Check sheet for the modelled part. Datum: model origin and axes. Units: mm. A direction names the side the tool comes from. Coordinates: 2 decimals unless noted, no trailing zeros. Loops run counter-clockwise (first coordinate to the right, second up) from the corner with the lowest first, then second, coordinate; pieces in that order, holes last.
```python
from build123d import *

# Parameters (mm, degrees)
SKETCH1_R                    = 254
BOSS_EXTRUDE1_DEPTH          = 2.54
SKETCH2_R                    = 228.6
SKETCH2_R_2                  = 226.06
CUT_EXTRUDE1_DEPTH           = 1.27
CUT_EXTRUDE2_DEPTH           = 1.27
SKETCH8_R                    = 6.35
CUT_EXTRUDE3_DEPTH           = 360.219224987
F_10_0_1935_DIAMETER_HOLE1_D = 4.9149


with BuildPart() as part:
    # Sketch1 → Boss-Extrude1 (new body)
    with BuildSketch(Plane.XY):
        Circle(SKETCH1_R)
    extrude(amount=BOSS_EXTRUDE1_DEPTH)

    # Sketch2 → Cut-Extrude1 (cut)
    with BuildSketch(Plane.XY.offset(2.54)):
        Circle(SKETCH2_R)
        Circle(SKETCH2_R_2, mode=Mode.SUBTRACT)
    extrude(amount=-CUT_EXTRUDE1_DEPTH, mode=Mode.SUBTRACT)

    # Sketch4 → Cut-Extrude2 (cut)
    with BuildSketch(Plane.XY.offset(2.54)):
        with BuildLine():
            Line((-226.06, 0), (-175.26, 18.489687901))
            Line((-175.26, 18.489687901), (-176.128731164, 20.876507158))
            Line((-176.128731164, 20.876507158), (-226.043768674, 2.708919262))
            ThreePointArc((-226.043768674, 2.708919262), (-226.055942132, 1.354483944), (-226.06, 0))
        make_face()
        with BuildLine():
            Line((-195.77370278, 113.03), (-142.534768317, 103.64253943))
            Line((-142.534768317, 103.64253943), (-142.093701946, 106.143951123))
            Line((-142.093701946, 106.143951123), (-194.405186408, 115.367877234))
            ThreePointArc((-194.405186408, 115.367877234), (-195.092946591, 114.200988571), (-195.77370278, 113.03))
        make_face()
        with BuildLine():
            Line((-113.03, 195.77370278), (-71.61746057, 161.024456218))
            Line((-71.61746057, 161.024456218), (-69.984780041, 162.970209103))
            Line((-69.984780041, 162.970209103), (-110.67589144, 197.11410567))
            ThreePointArc((-110.67589144, 197.11410567), (-111.854953561, 196.447430535), (-113.03, 195.77370278))
        make_face()
        with BuildLine():
            Line((0, 226.06), (18.489687901, 175.26))
            Line((18.489687901, 175.26), (20.876507158, 176.128731164))
            Line((20.876507158, 176.128731164), (2.708919262, 226.043768674))
            ThreePointArc((2.708919262, 226.043768674), (1.354483944, 226.055942132), (0, 226.06))
        make_face()
        with BuildLine():
            Line((113.03, 195.77370278), (103.64253943, 142.534768317))
            Line((103.64253943, 142.534768317), (106.143951123, 142.093701946))
            Line((106.143951123, 142.093701946), (115.367877234, 194.405186408))
            ThreePointArc((115.367877234, 194.405186408), (114.200988571, 195.092946591), (113.03, 195.77370278))
        make_face()
        with BuildLine():
            Line((195.77370278, 113.03), (161.024456218, 71.61746057))
            Line((161.024456218, 71.61746057), (162.970209103, 69.984780041))
            Line((162.970209103, 69.984780041), (197.11410567, 110.67589144))
            ThreePointArc((197.11410567, 110.67589144), (196.447430535, 111.854953561), (195.77370278, 113.03))
        make_face()
        with BuildLine():
            Line((226.06, 0), (175.26, -18.489687901))
            Line((175.26, -18.489687901), (176.128731164, -20.876507158))
            Line((176.128731164, -20.876507158), (226.043768674, -2.708919262))
            ThreePointArc((226.043768674, -2.708919262), (226.055942132, -1.354483944), (226.06, 0))
        make_face()
        with BuildLine():
            Line((195.77370278, -113.03), (142.534768317, -103.64253943))
            Line((142.534768317, -103.64253943), (142.093701946, -106.143951123))
            Line((142.093701946, -106.143951123), (194.405186408, -115.367877234))
            ThreePointArc((194.405186408, -115.367877234), (195.092946591, -114.200988571), (195.77370278, -113.03))
        make_face()
        with BuildLine():
            Line((113.03, -195.77370278), (71.61746057, -161.024456218))
            Line((71.61746057, -161.024456218), (69.984780041, -162.970209103))
            Line((69.984780041, -162.970209103), (110.67589144, -197.11410567))
            ThreePointArc((110.67589144, -197.11410567), (111.854953561, -196.447430535), (113.03, -195.77370278))
        make_face()
        with BuildLine():
            Line((0, -226.06), (-18.489687901, -175.26))
            Line((-18.489687901, -175.26), (-20.876507158, -176.128731164))
            Line((-20.876507158, -176.128731164), (-2.708919262, -226.043768674))
            ThreePointArc((-2.708919262, -226.043768674), (-1.354483944, -226.055942132), (0, -226.06))
        make_face()
        with BuildLine():
            Line((-113.03, -195.77370278), (-103.64253943, -142.534768317))
            Line((-103.64253943, -142.534768317), (-106.143951123, -142.093701946))
            Line((-106.143951123, -142.093701946), (-115.367877234, -194.405186408))
            ThreePointArc((-115.367877234, -194.405186408), (-114.200988571, -195.092946591), (-113.03, -195.77370278))
        make_face()
        with BuildLine():
            Line((-195.77370278, -113.03), (-161.024456218, -71.61746057))
            Line((-161.024456218, -71.61746057), (-162.970209103, -69.984780041))
            Line((-162.970209103, -69.984780041), (-197.11410567, -110.67589144))
            ThreePointArc((-197.11410567, -110.67589144), (-196.447430535, -111.854953561), (-195.77370278, -113.03))
        make_face()
    extrude(amount=-CUT_EXTRUDE2_DEPTH, mode=Mode.SUBTRACT)

    # Sketch8 → Cut-Extrude3 (cut, through all)
    with BuildSketch(Plane(origin=(0, 0, 0), x_dir=(-1, 0, 0), z_dir=(0, 0, -1))):
        Circle(SKETCH8_R)
    extrude(amount=-CUT_EXTRUDE3_DEPTH, mode=Mode.SUBTRACT)

    # #10 (0.1935) Diameter Hole1 (through all)
    with Locations(Plane.XY.offset(2.54)):
        with Locations((-235.585, 0), (-166.583751046, 166.583751046), (0, 235.585), (166.583751046, 166.583751046), (235.585, 0), (166.583751046, -166.583751046), (0, -235.585), (-166.583751046, -166.583751046)):
            Hole(F_10_0_1935_DIAMETER_HOLE1_D / 2)


solid = part.part
```
1) Section check C-C on y = -187. Enter the section's corners in (x, z), plus the area to 3 significant figures.
Answer sheet:
outline: (-171.89, 0) - (171.89, 0) - (171.89, 2.54) - (131.49, 2.54) - (131.49, 1.27) - (127.02, 1.27) - (127.02, 2.54) - (102.57, 2.54) - (102.57, 1.27) - (98.62, 1.27) - (98.62, 2.54) - (-14.22, 2.54) - (-14.22, 1.27) - (-16.92, 1.27) - (-16.92, 2.54) - (-111.48, 2.54) - (-111.48, 1.27) - (-114.06, 1.27) - (-114.06, 2.54) - (-127.02, 2.54) - (-127.02, 1.27) - (-131.49, 1.27) - (-131.49, 2.54) - (-171.89, 2.54) - close
area: 850 mm2
2) Section check A-A on z = 0.6. Give the number of separate pieces and of enclosed holes in the cut face, plus the area to 3 significant figures.
Answer sheet:
separate pieces: 1
enclosed holes: 9
area: 202,000 mm2
3) Section check B-B on y = 129.5. Enter the section's corners in (x, z).
Answer sheet:
outline: (-218.51, 0) - (218.51, 0) - (218.51, 2.54) - (188.38, 2.54) - (188.38, 1.27) - (185.29, 1.27) - (185.29, 2.54) - (-185.29, 2.54) - (-185.29, 1.27) - (-188.38, 1.27) - (-188.38, 2.54) - (-218.51, 2.54) - close
4) Depth check by flat-ended pin: pin 1 (4.5 mm diameter, centred on x = 235.585, y = 0, fed in from +Z). Enter the tip coordinate at first touch or a pass-through.
Answer sheet:
pin 1: passes through
5) Set-up check for faces 1 (the cylindrical face through (217.787, -60.596, 1.914)), 2 (the cylindrical face through (1.38, -6.2, 1.25)): record each of +Z, -Z, +X, -X, +Y, -Y from which the full face is reachable in a straight line by a thin tool's end or side.
Answer sheet:
face 1: +Z
face 2: +Z, -Z
6) Scan lines: line 1 (X direction, y = -67, z = 1.65); line 2 (Y direction, x = -195, z = 1.65); line 3 (Y direction, x = -174, z = 2). Record each from-to range of solid material in increasing order.
Answer sheet:
line 1: x = -245 to -218.56, -215.9 to 215.9, 218.56 to 245
line 2: y = -162.76 to -119.3, -114.36 to -112.11, -108.16 to 11.3, 14.01 to 112.89, 119.3 to 162.76
line 3: y = -185.04 to -148.26, -144.32 to -87.08, -83.13 to 109.19, 111.77 to 144.32, 148.26 to 185.04
